Check sheet for the modelled part. Datum: model origin and axes. Units: mm. A direction names the side the tool comes from. Round coordinates to 2 decimals unless told otherwise and drop trailing zeros. Order: outer loops, then holes, each group sorted by start corner. A loop starts at its lowest first (then second) coordinate and runs counter-clockwise, first axis right, second up.
(1) Thickness scan on probe 1 along Z at (x, y) = (40, 2); probe 2 along Z at (x, y) = (4, 2.5); probe 3 along X at (y, z) = (7, 9). Record the ranges inside material, lowest first.
(2) Depth check by flat-ended pin: pin 1 (2 mm diameter, centred on x = 40, z = -10, fed in from +Y); pin 2 (4 mm diameter, centred on x = 30.85, z = -4, fed in from -Y); pin 3 (1.5 mm diameter, centred on x = -30, z = -4.5, fed in from +Y); pin 4 (8 mm diameter, centred on x = 41, z = 6.5, fed in from +Y). Enter the tip coordinate at first touch or a pass-through.
(3) Mould release check, pull along X, two halves, no side actions. Record for faces 1 (the flat face through (0, 8, 12)), 2 (the flat face through (-45, 1, 0)), 3 (the flat face through (33.13, 12.06, -8.86)), 4 (the flat face through (-1, 4, 14)): released by +X, released by -X, zero draft, split by the parting line, or undercut.
(4) Sectioned sample at C-C, the plane z = -3.5. Enter the section's corners in (x, y).
(5) Sectioned sample at D-D, the plane y = 4. Enter the section's corners in (x, z).
(6) Tool access check on faces 5 (the flat face through (-31, 2, -4)), 6 (the flat face through (-18.85, 4, 0)), 7 (the flat face through (23.495, 12.056, 8.67)), 8 (the cylindrical face through (29.821, 11.944, -10.077)). Record the directions out of +Z, -Z, +X, -X, +Y, -Y that give a thin tool (end or side, any length) a straight path to the whole face; none if there is none.
(7) Sectioned sample at A-A, the plane y = 14.25. Enter the section's corners in (x, z), and give its area (3 significant figures).
(8) Sectioned sample at B-B, the plane x = -40. Enter the section's corners in (y, z), and give its area (3 significant figures).
```python
from build123d import *

# Parameters (mm, degrees)
SKETCH1_W                = 10.15
SKETCH1_H                = 28
SKETCH1_W_2              = 69.7
BOSS_EXTRUDE1_DEPTH      = 3
SKETCH1_3_W              = 69.7
SKETCH1_3_H              = 28
BOSS_EXTRUDE2_DEPTH      = 8
SKETCH2_R                = 2.5
CUT_EXTRUDE1_DEPTH       = 6
BOSS_EXTRUDE3_START      = -8
SKETCH3_R                = 2.5
BOSS_EXTRUDE3_DEPTH      = 8
FILLET1_R                = 2
FILLET1_OF_MIRROR1_R     = 2
M3_CLEARANCE_HOLE1_D     = 3.6
M3_CLEARANCE_HOLE1_DEPTH = 10
M3_CLEARANCE_HOLE1_TIP   = 1.081549114
SKETCH6_W                = 37.7
SKETCH6_H                = 20
CUT_EXTRUDE2_DEPTH       = 48.801673611


with BuildPart() as part:
    # Sketch1 → Boss-Extrude1 (new body)
    with BuildSketch(Plane(origin=(0, 0, 0), x_dir=(1, 0, 0), z_dir=(0, 1, 0))):
        with Locations((-39.925, 0)):
            Rectangle(SKETCH1_W, SKETCH1_H)
        Rectangle(SKETCH1_W_2, SKETCH1_H)
        with Locations((39.925, 0)):
            Rectangle(SKETCH1_W, SKETCH1_H)
    extrude(amount=BOSS_EXTRUDE1_DEPTH)

    # Sketch1<3> → Boss-Extrude2 (add)
    with BuildSketch(Plane(origin=(0, 0, 0), x_dir=(1, 0, 0), z_dir=(0, 1, 0))):
        Rectangle(SKETCH1_3_W, SKETCH1_3_H)
    extrude(amount=BOSS_EXTRUDE2_DEPTH)

    # Sketch2 → Cut-Extrude1 (cut)
    with BuildSketch(Plane.XZ.offset(-8)):
        with Locations(Location((-30.85, -4, 0), (0, 0, 90))):
            Circle(SKETCH2_R)
        with Locations(Location((-26.2, 4.054036255, 0), (0, 0, 90))):
            Circle(SKETCH2_R)
    cut_extrude1 = extrude(amount=CUT_EXTRUDE1_DEPTH, mode=Mode.SUBTRACT)

    # Sketch3 → Boss-Extrude3 (add)
    with BuildSketch(Plane.XZ.offset(-8).offset(BOSS_EXTRUDE3_START)):
        Polygon((-29.627885683, -10.88323591), (-19.627885683, 6.437272165), (-27.422114317, 10.937272165), (-34.85, -1.92820323), (-34.85, -7.868246804), align=None)
        with Locations(Location((-30.85, -4, 0), (0, 0, 90))):
            Circle(SKETCH3_R, mode=Mode.SUBTRACT)
        with Locations(Location((-26.2, 4.054036255, 0), (0, 0, 90))):
            Circle(SKETCH3_R, mode=Mode.SUBTRACT)
    boss_extrude3 = extrude(amount=BOSS_EXTRUDE3_DEPTH)

    # Fillet1
    fillet1_edges = [part.edges().sort_by_distance(p)[0] for p in [
        (-27.422114317, 12, 10.937272165),
        (-19.627885683, 12, 6.437272165),
        (-29.627885683, 12, -10.88323591),
    ]]
    fillet(fillet1_edges, radius=FILLET1_R)

    # Mirror1: Cut-Extrude1, Boss-Extrude3 across plane
    add(cut_extrude1.mirror(Plane(origin=(0, 0, 0), x_dir=(0, 0, 1), z_dir=(1, 0, 0))), mode=Mode.SUBTRACT)
    add(boss_extrude3.mirror(Plane(origin=(0, 0, 0), x_dir=(0, 0, 1), z_dir=(1, 0, 0))))

    # Fillet1 of Mirror1
    fillet1_of_mirror1_edges = [part.edges().sort_by_distance(p)[0] for p in [
        (27.422114317, 12, 10.937272165),
        (19.627885683, 12, 6.437272165),
        (29.627885683, 12, -10.88323591),
    ]]
    fillet(fillet1_of_mirror1_edges, radius=FILLET1_OF_MIRROR1_R)

    # M3 Clearance Hole1
    with Locations(Plane(origin=(0, 3, 0), x_dir=(1, 0, 0), z_dir=(0, 1, 0))):
        with Locations((-40, 10), (-40, -10), (40, -10), (40, 10)):
            Hole(M3_CLEARANCE_HOLE1_D / 2, depth=M3_CLEARANCE_HOLE1_DEPTH)
            with Locations((0, 0, -(M3_CLEARANCE_HOLE1_DEPTH + M3_CLEARANCE_HOLE1_TIP / 2))):  # 118° drill point
                Cone(0, M3_CLEARANCE_HOLE1_D / 2, M3_CLEARANCE_HOLE1_TIP, mode=Mode.SUBTRACT)

    # Sketch6 → Cut-Extrude2 (cut, through all)
    with BuildSketch(Plane(origin=(0, 8, 0), x_dir=(1, 0, 0), z_dir=(0, 1, 0))):
        Rectangle(SKETCH6_W, SKETCH6_H)
    extrude(amount=-CUT_EXTRUDE2_DEPTH, mode=Mode.SUBTRACT)


solid = part.part
```
Derived:
1. probe 1: z = -14 to -11.8, -8.2 to 8.2, 11.8 to 14
1. probe 2: z = -14 to -10, 10 to 14
1. probe 3: x = -34.85 to -18.85, 18.85 to 34.85
2. pin 1: passes through
2. pin 2: stops at y = 0
2. pin 3: stops at y = 2
2. pin 4: stops at y = 3
3. face 1: undercut
3. face 2: released by -X
3. face 3: released by +X
3. face 4: zero draft
4. outline: (-45, 0) - (-18.85, 0) - (-18.85, 8) - (-25.37, 8) - (-25.37, 16) - (-28.4, 16) - (-28.4, 2) - (-33.3, 2) - (-33.3, 16) - (-34.85, 16) - (-34.85, 3) - (-45, 3) - close; (18.85, 0) - (45, 0) - (45, 3) - (34.85, 3) - (34.85, 16) - (33.3, 16) - (33.3, 2) - (28.4, 2) - (28.4, 16) - (25.37, 16) - (25.37, 8) - (18.85, 8) - close
5. outline: (-34.85, -14) - (34.85, -14) - (34.85, 14) - (-34.85, 14) - close; hole circle Ø5 at (-30.85, -4); hole circle Ø5 at (-26.2, 4.05); hole (-18.85, -10) - (18.85, -10) - (18.85, 10) - (-18.85, 10) - close; hole circle Ø5 at (26.2, 4.05); hole circle Ø5 at (30.85, -4)
6. face 5: +Y
6. face 6: +Y, -Y
6. face 7: +Z, +Y
6. face 8: -Z, +Y
7. outline: (-34.85, -7.87) - (-31.36, -9.88) arc R2 ccw to (-28.63, -9.15) - (-20.63, 4.71) arc R2 ccw to (-21.36, 7.44) - (-25.69, 9.94) arc R2 ccw to (-28.42, 9.21) - (-34.85, -1.93) - close; (20.63, 4.71) - (28.63, -9.15) arc R2 ccw to (31.36, -9.88) - (34.85, -7.87) - (34.85, -1.93) - (28.42, 9.21) arc R2 ccw to (25.69, 9.94) - (21.36, 7.44) arc R2 ccw to start; hole circle Ø5 at (-30.85, -4); hole circle Ø5 at (-26.2, 4.05); hole circle Ø5 at (26.2, 4.05); hole circle Ø5 at (30.85, -4)
7. area: 261 mm2
8. outline: (0, -14) - (3, -14) - (3, -11.8) - (0, -11.8) - close; (0, -8.2) - (3, -8.2) - (3, 8.2) - (0, 8.2) - close; (0, 11.8) - (3, 11.8) - (3, 14) - (0, 14) - close
8. area: 62.4 mm2
